Input: part model. Units: mm. Frame: model coordinates. A direction names the side the tool comes from. Give positions to 0.01 mm unless a question says otherwise; leave off trailing zeros. Loops run counter-clockwise (first coordinate to the right, second up) from the corner with the lowest first, then second, coordinate; pieces in that order, holes last. Notation, with made-up numbers: (0, -20.5) - (20, -20.5) arc R22 ccw to (20, -14.5) - close; hole circle Ø5 at (11.25, 88). An arc over 180 degrees is marked (long way). Answer as a JSON object with one key per item and string values.
from build123d import *

# Parameters (mm, degrees)
F0_W      = 27
F0_H      = 6.5
F1_DEPTH  = 25
F2_T      = -1
F3_W      = 9.5
F3_H      = 18
F4_DEPTH  = 1
F5_W      = 1
F5_H      = 22
F6_DEPTH  = 1
F7_W      = 3
F7_H      = 3
F8_DEPTH  = 2
F9_W      = 2
F9_H      = 3
F9_W_2    = 3
F10_DEPTH = 1.5


with BuildPart() as f1:
    # F0 (on Top) → F1 (new body)
    with BuildSketch(Plane.XY):
        with Locations((13.5, 3.25)):
            Rectangle(F0_W, F0_H)
    extrude(amount=F1_DEPTH)

    # F2
    f2_openings = [f1.faces().sort_by_distance(p)[0] for p in [
        (13.5, 3.25, 25),
    ]]
    offset(amount=F2_T, openings=f2_openings)

    # F3 (on face) → F4 (cut, through all)
    with BuildSketch(Plane.XZ):
        with Locations((10.75, 16)):
            Rectangle(F3_W, F3_H)
    extrude(amount=-F4_DEPTH, mode=Mode.SUBTRACT)

    # F5 (on face) → F6 (cut, through all)
    with BuildSketch(Plane(origin=(0, 0, 0), x_dir=(0, -1, 0), z_dir=(-1, 0, 0))):
        with Locations((-4, 14)):
            Rectangle(F5_W, F5_H)
    extrude(amount=-F6_DEPTH, mode=Mode.SUBTRACT)

    # F7 (on face) → F8 (join)
    with BuildSketch(Plane(origin=(0, 6.5, 0), x_dir=(-1, 0, 0), z_dir=(0, 1, 0))):
        with Locations((-13.5, 1.5)):
            Rectangle(F7_W, F7_H)
    extrude(amount=F8_DEPTH)

    # F9 (on face) → F10 (join)
    with BuildSketch(Plane(origin=(0, 8.5, 0), x_dir=(-1, 0, 0), z_dir=(0, 1, 0))):
        with Locations((-11, 1.5)):
            Rectangle(F9_W, F9_H)
        with Locations((-13.5, 1.5)):
            Rectangle(F9_W_2, F9_H)
        with Locations((-16, 1.5)):
            Rectangle(F9_W, F9_H)
    extrude(amount=F10_DEPTH)


solid = f1.part
Item 1: Cut plane B-B (z = 12). Return loops of the section in (x, y), then the cut area to 3 significant figures.
Geometry check:
{"outline": "(0, 0) - (6, 0) - (6, 1) - (1, 1) - (1, 3.5) - (0, 3.5) - close; (0, 4.5) - (1, 4.5) - (1, 5.5) - (26, 5.5) - (26, 1) - (15.5, 1) - (15.5, 0) - (27, 0) - (27, 6.5) - (0, 6.5) - close", "area": "52.5 mm2"}
Item 2: Cut plane D-D (y = 1.75). Return loops of the section in (x, z), then the cut area to 3 significant figures.
Geometry check:
{"outline": "(0, 0) - (27, 0) - (27, 25) - (26, 25) - (26, 1) - (1, 1) - (1, 25) - (0, 25) - close", "area": "75.0 mm2"}
Item 3: Cut plane C-C (z = 2.25). Return loops of the section in (x, y).
Geometry check:
{"outline": "(0, 0) - (27, 0) - (27, 6.5) - (15, 6.5) - (15, 8.5) - (17, 8.5) - (17, 10) - (10, 10) - (10, 8.5) - (12, 8.5) - (12, 6.5) - (0, 6.5) - close; hole (1, 1) - (26, 1) - (26, 5.5) - (1, 5.5) - close"}
Item 4: Access query for faces 4 (the face through (17, 9, 1)), 5 (the face through (15, 7, 1)), 6 (the face through (0.5, 3.5, 13.8)), 7 (the face through (1, 3, 13)), 8 (the face through (12, 7, 1)). Directions: +Z, -Z, +X, -X, +Y, -Y. A direction counts if a zero-diameter tool reaches every point of the face in a straight line with its end or side. Return the directions, or none.
Geometry check:
{"face 4": "+Z, -Z, +X, +Y", "face 5": "+Z, -Z, +X", "face 6": "+Z, -X", "face 7": "+Z", "face 8": "+Z, -Z, -X"}
Item 5: Contact query for flat-ended pins moving along their axis: P1, Ø1, axis at y = 7.5, z = 1.5, coming from the +X side; P2, Ø1, axis at x = 10, z = 14.5, coming from the +Y side; P3, Ø0.8, axis at x = 11.5, y = 0.5, coming from the +Z side. Output: stop coordinate, or through.
Geometry check:
{"P1": "stops at x = 15", "P2": "stops at y = 6.5", "P3": "stops at z = 7"}
Item 6: Material intervals for line 1 (Y direction, x = 10.75, z = 1.75); line 2 (X direction, y = 2, z = 20.25); line 3 (Y direction, x = 18, z = 19.75), sorted ascending. Write a range as [from, to].
Geometry check:
{"line 1": "y = [0, 1], [5.5, 6.5], [8.5, 10]", "line 2": "x = [0, 1], [26, 27]", "line 3": "y = [0, 1], [5.5, 6.5]"}
Item 7: Mould query, pull axis X, two halves, no side actions, for faces 1 (the face through (10, 9, 1)), 2 (the face through (15.5, 0.5, 15.9)), 3 (the face through (16, 8.5, 2)). Classes: released by +X, released by -X, zero draft, split by the parting line, or undercut.
Geometry check:
{"face 1": "released by -X", "face 2": "undercut", "face 3": "zero draft"}
Item 8: Cut plane A-A (x = 16). Return loops of the section in (y, z).
Geometry check:
{"outline": "(0, 0) - (6.5, 0) - (6.5, 25) - (5.5, 25) - (5.5, 1) - (1, 1) - (1, 25) - (0, 25) - close; (8.5, 0) - (10, 0) - (10, 3) - (8.5, 3) - close"}
